from build123d import *

# Parameters (mm, degrees)
SKETCH002_W  = 77.5
SKETCH002_H  = 77.5
SKETCH002_R  = 1.85
PAD_DEPTH    = 5.7
FILLET_R     = 5
SKETCH_R     = 32.537283
POCKET_DEPTH = 5.7


with BuildPart() as part:
    # Sketch001 → Revolution (revolve)
    with BuildSketch(Plane.XZ):
        with BuildLine():
            Line((0, 41.745886), (0, 74.590784))
            Line((0, 74.590784), (26.5, 74.590784))
            Line((26.5, 74.590784), (26.5, 53.340784))
            Line((26.5, 53.340784), (36.5, 32.090784))
            Line((36.5, 32.090784), (33.5, 32.090784))
            Line((33.5, 32.090784), (10, 46.745886))
            add(Edge.make_bspline(
                [(0, 41.745886), (8.313298, 41.745886), (10, 46.745886)],
                knots=[1.570796, 1.570796, 1.570796, 2.937282, 2.937282, 2.937282], degree=2, weights=[1, 0.77553, 1]))
        make_face()
    revolve(axis=Axis((0, 0, 0), (0, 0, 1)))

    # Sketch002 → Pad (new body)
    with BuildSketch(Plane(origin=(0, 0, 31.993353), x_dir=(1, 0, 0), z_dir=(0, 0, -1))):
        Rectangle(SKETCH002_W, SKETCH002_H)
        with Locations((-31.819805, 31.819805)):
            Circle(SKETCH002_R, mode=Mode.SUBTRACT)
        with Locations((31.819805, 31.819805)):
            Circle(SKETCH002_R, mode=Mode.SUBTRACT)
        with Locations((-31.819805, -31.819805)):
            Circle(SKETCH002_R, mode=Mode.SUBTRACT)
        with Locations((31.819805, -31.819805)):
            Circle(SKETCH002_R, mode=Mode.SUBTRACT)
    extrude(amount=-PAD_DEPTH)

    # Fillet
    fillet_edges = [part.edges().sort_by_distance(p)[0] for p in [
        (38.75, -38.75, 34.843353),
        (-38.75, -38.75, 34.843353),
        (-38.75, 38.75, 34.843353),
        (38.75, 38.75, 34.843353),
    ]]
    fillet(fillet_edges, radius=FILLET_R)

    # Sketch → Pocket (cut)
    with BuildSketch(Plane(origin=(0, 0, 31.993353), x_dir=(1, 0, 0), z_dir=(0, 0, -1))):
        Circle(SKETCH_R)
    extrude(amount=-POCKET_DEPTH, mode=Mode.SUBTRACT)


solid = part.part
The listing builds one solid part. Answer for the finished solid, in the listing's coordinates (mm). A direction names the side the tool comes from. Give positions to 0.01 mm unless a question says otherwise; leave off trailing zeros. Write each loop counter-clockwise with the first axis right and the second up, starting at its lowest first coordinate (ties: lowest second). Pieces come first, ordered by that corner, then holes. Notation, with made-up numbers: (18.25, -13) - (76.25, -13) arc R33 cw to (76.25, 18) - close; hole circle Ø5 at (43, -25). An arc over 180 degrees is marked (long way). Use a Markdown table: item, result.
1. A tool of negligible diameter and unlimited length cuts with its end or side. For faces 4 (the flat face through (38.75, 0, 35)), 5 (the cylindrical face through (-32.506, -1.431, 34.803)), 6 (the flat face through (-35, -1, 37.693)), from which of +Z, -Z, +X, -X, +Y, -Y can it reach the whole face along a straight path? Write none if from no direction.
Values follow:
| item | result |
|---|---|
| face 4 | +Z, -Z, +X, +Y, -Y |
| face 5 | -Z |
| face 6 | +Z |
2. For a pull along Y with two mould halves and no side action, classify faces 1 (the flat face through (0, -38.75, 35)), 2 (the cylindrical face through (14.246, 22.345, 63.817)), 3 (the cylindrical face through (31.579, 29.986, 34.803)) as released by +Y, released by -Y, zero draft, split by the parting line, or undercut.
Values follow:
| item | result |
|---|---|
| face 1 | released by -Y |
| face 2 | split by the parting line |
| face 3 | undercut |
3. Section B-B on z = 52 is taken. Write down the section's boundary in (x, y).
Values follow:
| item | result |
|---|---|
| outline | circle Ø54.26 at (0, 0) |
4. Section A-A on z = 58 is taken. Write down the section's boundary in (x, y), plus the area to 3 significant figures.
Values follow:
| item | result |
|---|---|
| outline | circle Ø53 at (0, 0) |
| area | 2,210 mm² |
5. Each of these flat-tipped pins is pushed along its axis until it touches: P1, Ø12, axis at x = -17.5, z = 47.5, coming from the -Y side; P2, Ø3, axis at x = 12.5, y = 20.5, coming from the -Z side; P3, Ø10, axis at x = -4.5, y = 5, coming from the -Z side. Where does it stop, or does it pass through?
Values follow:
| item | result |
|---|---|
| P1 | stops at y = -28.3 |
| P2 | stops at z = 37.69 |
| P3 | stops at z = 41.84 |
6. Find the intervals of material crossed by probe 1 along Y at (x, z) = (-4, 46.5); probe 2 along X at (y, z) = (2, 38); probe 3 along Z at (x, y) = (23, -35), in increasing order. Write a range as from..to.
Values follow:
| item | result |
|---|---|
| probe 1 | y = -29.45..-9.59, -9.07..9.07, 9.59..29.45 |
| probe 2 | x = -33.66..-23.94, 23.94..33.66 |
| probe 3 | z = 31.99..37.69 |
